```python
from build123d import *

# Parameters (mm, degrees)
SKETCH1_W           = 38
SKETCH1_H           = 38
BOSS_EXTRUDE1_DEPTH = 4
BOSS_EXTRUDE2_DEPTH = 2
FILLET1_R           = 3


with BuildPart() as part:
    # Sketch1 → Boss-Extrude1 (new body)
    with BuildSketch(Plane(origin=(0, 0, 0), x_dir=(1, 0, 0), z_dir=(0, 1, 0))):
        Rectangle(SKETCH1_W, SKETCH1_H)
    extrude(amount=BOSS_EXTRUDE1_DEPTH)

    # Sketch2 → Boss-Extrude2 (add)
    with BuildSketch(Plane(origin=(0, 4, 0), x_dir=(1, 0, 0), z_dir=(0, 1, 0))):
        Polygon((-16, -19), (-19, -19), (-19, 19), (19, 19), (19, 16), (-16, 16), align=None)
    extrude(amount=BOSS_EXTRUDE2_DEPTH)

    # Fillet1
    fillet1_edges = [part.edges().sort_by_distance(p)[0] for p in [
        (-19, 3, -19),
    ]]
    fillet(fillet1_edges, radius=FILLET1_R)


solid = part.part
```
Verification items for the finished model (mm, model axes). A direction names the side the tool comes from. Round coordinates to 2 decimals unless told otherwise and drop trailing zeros. Order: outer loops, then holes, each group sorted by start corner. A loop starts at its lowest first (then second) coordinate and runs counter-clockwise, first axis right, second up. Notation, with made-up numbers: (-6.5, 6) - (13.5, 6) arc R13 ccw to (13.5, 26) - close; hole circle Ø7 at (1.5, 26). An arc over 180 degrees is marked (long way). Use CSV: the item, a comma, the result in double quotes. Start each with the question number.
1) Access from +Z, -Z, +X, -X, +Y, -Y to the whole of each face (thin tool, end or side, straight path). Record for faces 1 (the flat face through (-16, 5, 1)), 2 (the flat face through (0, 0, 0)).
2) Section check B-B, the plane z = 9. Record the cut outline in (x, y).
3) Section check A-A, the plane y = 4.6. Record the cut outline in (x, z).
4) Go/stop test with flat-tipped pins: P1, Ø1.5, axis at x = 2, z = 6.5, coming from the +Y side; P2, Ø1, axis at y = 5, z = -2, coming from the +X side. Record where each tip stops, or that it passes through.
5) Section check C-C, the plane x = 16. Record the cut outline in (y, z), plus the area to 3 significant figures.
6) Thickness scan on L1, parallel to Y at x = -14, z = 17; L2, parallel to Z at x = 1, y = 4.4. Record the ranges inside material, lowest first.
Answers:
1,face 1,"+Z, +X, +Y"
1,face 2,"+Z, -Z, +X, -X, -Y"
2,outline,"(-19, 0) - (19, 0) - (19, 4) - (-16, 4) - (-16, 6) - (-19, 6) - close"
3,outline,"(-19, -16) arc R3 ccw to (-16, -19) - (19, -19) - (19, -16) - (-16, -16) - (-16, 19) - (-19, 19) - close"
4,P1,"stops at y = 4"
4,P2,"stops at x = -16"
5,outline,"(0, -19) - (6, -19) - (6, -16) - (4, -16) - (4, 19) - (0, 19) - close"
5,area,"158 mm²"
6,L1,"y = 0 to 4"
6,L2,"z = -19 to -16"
